```python
from build123d import *

# Parameters (mm, degrees)
BOSS_EXTRUDE1_DEPTH = 3
FILLET1_R           = 0.2


with BuildPart() as part:
    # Sketch1 → Boss-Extrude1 (new body)
    with BuildSketch(Plane(origin=(0, 0, 0), x_dir=(1, 0, 0), z_dir=(0, 1, 0))):
        with BuildLine():
            Line((-25, 8.667504193), (-25, 31))
            ThreePointArc((-25, 31), (-24.414213562, 32.414213562), (-23, 33))
            Line((-23, 33), (-21, 33))
            Line((-21, 33), (-21, 21))
            ThreePointArc((-21, 21), (-17.75, 17.75), (-14.5, 21))
            Line((-14.5, 21), (-14.5, 34))
            ThreePointArc((-14.5, 34), (-13.914213562, 35.414213562), (-12.5, 36))
            Line((-12.5, 36), (12.5, 36))
            ThreePointArc((12.5, 36), (13.914213562, 35.414213562), (14.5, 34))
            Line((14.5, 34), (14.5, 21))
            ThreePointArc((14.5, 21), (17.75, 17.75), (21, 21))
            Line((21, 21), (21, 33))
            Line((21, 33), (23, 33))
            ThreePointArc((23, 33), (24.414213562, 32.414213562), (25, 31))
            Line((25, 31), (25, 8.667504193))
            ThreePointArc((25, 8.667504193), (23.791296457, 5.0559286), (20.652173913, 2.899461079))
            ThreePointArc((20.652173913, 2.899461079), (0, 0), (-20.652173913, 2.899461079))
            ThreePointArc((-20.652173913, 2.899461079), (-23.791296457, 5.0559286), (-25, 8.667504193))
        make_face()
    extrude(amount=BOSS_EXTRUDE1_DEPTH)

    # Fillet1
    fillet1_edges = [part.edges().sort_by_distance(p)[0] for p in [
        (-22, 3, -33),
        (-24.414213562, 3, -32.414213562),
        (-14.5, 0, -27.5),
        (-25, 3, -19.833752096),
        (-13.914213562, 0, -35.414213562),
        (0, 0, -36),
        (13.914213562, 0, -35.414213562),
        (14.5, 0, -27.5),
        (17.75, 0, -17.75),
        (21, 0, -27),
        (22, 0, -33),
        (24.414213562, 0, -32.414213562),
        (-23.791296457, 3, -5.0559286),
        (25, 0, -19.833752096),
        (23.791296457, 0, -5.0559286),
        (0, 0, 0),
        (-23.791296457, 0, -5.0559286),
        (-25, 0, -19.833752096),
        (-24.414213562, 0, -32.414213562),
        (-22, 0, -33),
        (0, 3, 0),
        (-21, 0, -27),
        (-17.75, 0, -17.75),
        (23.791296457, 3, -5.0559286),
        (25, 3, -19.833752096),
        (24.414213562, 3, -32.414213562),
        (22, 3, -33),
        (21, 3, -27),
        (-17.75, 3, -17.75),
        (17.75, 3, -17.75),
        (14.5, 3, -27.5),
        (13.914213562, 3, -35.414213562),
        (0, 3, -36),
        (-13.914213562, 3, -35.414213562),
        (-14.5, 3, -27.5),
        (-21, 3, -27),
    ]]
    fillet(fillet1_edges, radius=FILLET1_R)


solid = part.part
```
Verification items for the finished model (mm, model axes). A direction names the side the tool comes from. Give positions to 0.01 mm unless a question says otherwise; leave off trailing zeros. Order: outer loops, then holes, each group sorted by start corner. A loop starts at its lowest first (then second) coordinate and runs counter-clockwise, first axis right, second up. Notation, with made-up numbers: (-21, 30.25) -> (1, 30.25) arc R19 ccw to (1, 57.25) -> close; hole circle Ø6 at (-7.75, 9). An arc over 180 degrees is marked (long way). Use a Markdown table: item, result.
1) Material ranges on probe 1 along X at (y, z) = (1.4, -23.5); probe 2 along X at (y, z) = (1.7, -8.5); probe 3 along X at (y, z) = (0.85, -19), recorded low to high.
Results:
| item | result |
|---|---|
| probe 1 | -25 to -21, -14.5 to 14.5, 21 to 25 |
| probe 2 | -25 to 25 |
| probe 3 | -25 to -20.31, -15.19 to 15.19, 20.31 to 25 |
2) Mould release check, pull along X, two halves, no side actions. Record for faces 1 (the flat face through (-14.5, 1, -27)), 2 (the cylindrical face through (23.824, 1.482, -5.099)), 3 (the flat face through (-25, 1, -20)), 4 (the cylindrical face through (0, 1, 0)): pulls with the +X half, pulls with the -X half, needs draft (parallel to the pull), parting line crosses it, or undercut.
Results:
| item | result |
|---|---|
| face 1 | undercut |
| face 2 | pulls with the +X half |
| face 3 | pulls with the -X half |
| face 4 | parting line crosses it |
3) Tool access check on faces 5 (the flat face through (22, 1, -33)), 6 (the flat face through (-22, 1, -33)), 7 (the cylindrical face through (-23.758, 1.482, -5.013)), 8 (the flat face through (0, 0, -18)), 9 (the flat face through (-21, 1, -27)). Record the directions out of +Z, -Z, +X, -X, +Y, -Y that give a thin tool (end or side, any length) a straight path to the whole face; none if there is none.
Results:
| item | result |
|---|---|
| face 5 | -Z, +X, +Y, -Y |
| face 6 | -Z, -X, +Y, -Y |
| face 7 | +Z, -X, +Y, -Y |
| face 8 | +Z, -Z, +X, -X, -Y |
| face 9 | -Z, +Y, -Y |
4) Section check A-A, the plane z = -21.5. Record the boundary of the cut face in (x, y).
Results:
| item | result |
|---|---|
| outline | (-25, 0.2) arc R0.2 ccw to (-24.8, 0) -> (-21.2, 0) arc R0.2 ccw to (-21, 0.2) -> (-21, 2.8) arc R0.2 ccw to (-21.2, 3) -> (-24.8, 3) arc R0.2 ccw to (-25, 2.8) -> close; (-14.5, 0.2) arc R0.2 ccw to (-14.3, 0) -> (14.3, 0) arc R0.2 ccw to (14.5, 0.2) -> (14.5, 2.8) arc R0.2 ccw to (14.3, 3) -> (-14.3, 3) arc R0.2 ccw to (-14.5, 2.8) -> close; (21, 0.2) arc R0.2 ccw to (21.2, 0) -> (24.8, 0) arc R0.2 ccw to (25, 0.2) -> (25, 2.8) arc R0.2 ccw to (24.8, 3) -> (21.2, 3) arc R0.2 ccw to (21, 2.8) -> close |
5) Depth check by flat-ended pin: pin 1 Ø1 at (x, y) = (22.5, 1) entering from -Z; pin 2 Ø1.5 at (y, z) = (1.5, -31.5) entering from -X. Enter the tip coordinate at first touch or a pass-through.
Results:
| item | result |
|---|---|
| pin 1 | z = -33 |
| pin 2 | x = -25 |
6) Section check B-B, the plane y = 1. Record the boundary of the cut face in (x, z), then the cut area to 3 significant figures.
Results:
| item | result |
|---|---|
| outline | (-25, -31) arc R2 ccw to (-23, -33) -> (-21, -33) -> (-21, -21) arc R3.25 cw to (-14.5, -21) -> (-14.5, -34) arc R2 ccw to (-12.5, -36) -> (12.5, -36) arc R2 ccw to (14.5, -34) -> (14.5, -21) arc R3.25 cw to (21, -21) -> (21, -33) -> (23, -33) arc R2 ccw to (25, -31) -> (25, -8.67) arc R6 ccw to (20.65, -2.9) arc R75 ccw to (-20.65, -2.9) arc R6 ccw to (-25, -8.67) -> close |
| area | 1,470 mm² |
